```python
from build123d import *

# Parameters (mm, degrees)
F0_W     = 30
F0_H     = 100
F0_R     = 2.5
F0_W_2   = 17
F0_H_2   = 60
F1_DEPTH = 11
F2_R     = 2
F3_SIZE  = 1.5


with BuildPart() as f1:
    # F0 (on Top) → F1 (new body)
    with BuildSketch(Plane.XY):
        with Locations((5.474986, 0)):
            Rectangle(F0_W, F0_H)
        with Locations((5.474986, -40)):
            Circle(F0_R, mode=Mode.SUBTRACT)
        with Locations((5.474986, -0.691212)):
            Rectangle(F0_W_2, F0_H_2, mode=Mode.SUBTRACT)
        with Locations((5.474986, 40)):
            Circle(F0_R, mode=Mode.SUBTRACT)
    extrude(amount=F1_DEPTH)

    # F2
    f2_edges = [f1.edges().sort_by_distance(p)[0] for p in [
        (5.474986, 50, 11),
        (-9.525014, 0, 11),
        (20.474986, 0, 11),
        (5.474986, -50, 11),
        (-9.525014, -50, 5.5),
        (20.474986, -50, 5.5),
        (-9.525014, 50, 5.5),
        (20.474986, 50, 5.5),
        (13.974986, -0.691212, 11),
        (5.474986, -30.691212, 11),
        (-3.025014, -0.691212, 11),
        (5.474986, 29.308788, 11),
    ]]
    fillet(f2_edges, radius=F2_R)

    # F3
    f3_edges = [f1.edges().sort_by_distance(p)[0] for p in [
        (2.974986, 40, 11),
        (2.974986, -40, 11),
    ]]
    chamfer(f3_edges, length=F3_SIZE)


solid = f1.part
```
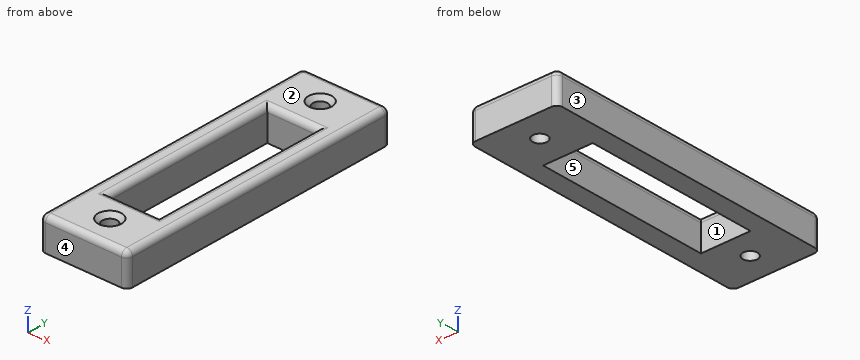
Could you check a few things on this model? Use its own coordinates, in mm. Face numbers are marked on the shaded views. A direction names the side the tool comes from. Round coordinates to 2 decimals unless told otherwise and drop trailing zeros. Write each loop counter-clockwise with the first axis right and the second up, starting at its lowest first coordinate (ties: lowest second). Pieces come first, ordered by that corner, then holes. Notation, with made-up numbers: M 38.25,-14 L 53.25,-14 A22 ccw 53.25,15 Z; hole C 33.5,63.5 d8. An arc over 180 degrees is marked long. Write each question's results on one line, items separated by ' | '. Start each with the question number.
1. Imagine slicing it at B-B on z = 7.5. List the corners of the cut face in (x, y) for me, and give its area (3 significant figures).
2. I need wall thicknesses on L1, parallel to X at y = 28.5, z = 8; L2, parallel to Y at x = 12.25, z = 6; L3, parallel to X at y = -41.5, z = 5.25. Which ranges of each line are inside material? Lowest first, please. Write a range as from..to.
3. Imagine slicing it at A-A on y = -19.5. List the corners of the cut face in (x, z) for me, and give its area (3 significant figures).
4. Imagine slicing it at D-D on x = 6.25. Count the separate pieces of the cut face and the enclosed holes in it, and give its area (3 significant figures).
5. Imagine slicing it at C-C on y = 40. List the corners of the cut face in (x, z) for me.
6. I'm going to push flat-ended pins straight in: pin 1 Ø3 at (x, y) = (5.47, -40) entering from +Z; pin 2 Ø8 at (x, y) = (-5.5, 18.5) entering from -Z; pin 3 Ø6 at (x, y) = (5.47, 40) entering from +Z (3 decimals). Where does each tip first touch, or does it pass through?
7. On a 3-axis mill with a long thin cutter (end or side, diameter ignored), from which of +Z, -Z, +X, -X, +Y, -Y can I reach the whole of each face in a straight line? I mean the marked faces 1 and 2. Say none if no direction works.
8. Thinking about a two-plate mould opening in X: for the marked faces 3, 4 and 5, which applies, +X half, -X half, draft (parallel to the pull), parting line (faces both ways), or undercut?
Result sheet:
1) outline: M -9.53,-48 A2 ccw -7.53,-50 L 18.47,-50 A2 ccw 20.47,-48 L 20.47,48 A2 ccw 18.47,50 L -7.53,50 A2 ccw -9.53,48 Z; hole M -3.03,-30.69 L 13.97,-30.69 L 13.97,29.31 L -3.03,29.31 Z; hole C 5.47,-40 d5; hole C 5.47,40 d5 | area: 1,940 mm^2
2) L1: x = -9.53..-3.03, 13.97..20.47 | L2: y = -50..-30.69, 29.31..50 | L3: x = -9.53..3.47, 7.47..20.47
3) outline: M -9.53,0 L -3.03,0 L -3.03,9 A2 ccw -5.03,11 L -7.53,11 A2 ccw -9.53,9 Z; M 13.97,0 L 20.47,0 L 20.47,9 A2 ccw 18.47,11 L 15.97,11 A2 ccw 13.97,9 Z | area: 140 mm^2
4) separate pieces: 4 | enclosed holes: 0 | area: 327 mm^2
5) outline: M -9.53,0 L 2.97,0 L 2.97,9.5 L 1.47,11 L -7.53,11 A2 ccw -9.53,9 Z; M 7.97,0 L 20.47,0 L 20.47,9 A2 ccw 18.47,11 L 9.47,11 L 7.97,9.5 Z
6) pin 1: passes through | pin 2: stops at z = 0 | pin 3: stops at z = 10.005
7) face 1: +Z, -Z | face 2: +Z, +X, -X, +Y, -Y
8) face 3: -X half | face 4: draft | face 5: undercut
